Model file for the job. Use its own axes, mm. A direction names the side the tool comes from. Round coordinates to 2 decimals unless told otherwise and drop trailing zeros. Write each loop counter-clockwise with the first axis right and the second up, starting at its lowest first coordinate (ties: lowest second). Pieces come first, ordered by that corner, then holes. Notation, with made-up numbers: (52.5, -33.75) - (70.5, -33.75) arc R18 ccw to (70.5, -9.75) - close; hole circle Ø3 at (-1.75, 61.25). An arc over 180 degrees is marked (long way). Answer as a JSON object with one key per item and string values. Group by question number.
Autodesk Inventor part; units mm, degrees
ref_plane "YZ Plane" through (0, 0, 0) normal (1, 0, 0) x (0, 1, 0)
ref_plane "XZ Plane" through (0, 0, 0) normal (0, 1, 0) x (-1, 0, 0)
ref_plane "XY Plane" through (0, 0, 0) normal (0, 0, 1) x (1, 0, 0)
sketch "Sketch1" plane through (0, 0, 0) normal (0, 1, 0) x (-1, 0, 0)
  line L0 (-40, 30) -> (40, 30)
  line L1 (40, 30) -> (40, -30)
  line L2 (40, -30) -> (-40, -30)
  line L3 (-40, -30) -> (-40, 30)
  line L4 (-40, 30) -> (40, -30) construction
  line L5 (40, 30) -> (-40, -30) construction
  line L6 (25.245, -30) -> (20.245, -30)
  line L7 (20.245, 30) -> (25.245, 30)
  line L8 (37, 30) -> (37, -30)
  line L9 (30.9, -30) -> (30.9, 30)
  line L10 (25.9, -30) -> (25.9, 30)
  line L11 (-10.1, -30) -> (-10.1, 30) construction
  point P0 (0, 0)
  point P1 (-35, 20)
  point P2 (-35, -20)
  point P3 (-20.1, 20)
  point P4 (-20.1, -20)
  dimension "d0" = 80
  dimension "d1" = 60
  dimension "d3" = 3
  dimension "d4" = 6.1
  dimension "d5" = 5
  dimension "d6" = 10
  dimension "d7" = 10
  dimension "d8" = 5
  dimension "d9" = 5
  dimension "d10" = 36
  dimension "d11" = 10
  dimension "d12" = 10
extrude "Extrusion1" add sketch "Sketch1" along normal blind 5
extrude "Extrusion2" add sketch "Sketch1" along normal blind 15 contours L0 L9 L2 L10 | L0 L1 L2 L8
chamfer "Chamfer1" distance 1 angle 45 2 edges at (-37, 15, 0) (-30.9, 15, 0)
fillet "Fillet1" radius 5 1 edges at (-25.9, 5, 0)
hole "Hole1" at (35, 0, 20) at (35, 0, -20) at (20.1, 0, 20) at (20.1, 0, -20) direction (0, 1, 0) diameter 3 end through all countersink diameter 6 countersink angle 90
properties part number "stabilisateur"
(1) Slice it at C-C (z = 20). Write the cut outline in (x, y), then the cut area to 3 significant figures.
(2) Drill centre lines: line 1 (X direction, y = 3.05, z = -20); line 2 (Z direction, x = 35, y = 3.35); line 3 (X direction, y = 14, z = -7.5). Where is each one in solid material? Low to high. Write a range as from..to.
(3) Flat gauge pins, fed straight in: pin 1 (1.8 mm diameter, centred on x = 35, z = -20, fed in from +Y); pin 2 (4 mm diameter, centred on y = 13.5, z = 6, fed in from +X); pin 3 (2 mm diameter, centred on x = 15.5, z = -22, fed in from +Y); pin 4 (5 mm diameter, centred on x = -30.5, z = 5.5, fed in from +Y). Where does each tip first touch, or does it go through?
(4) 3-axis set-ups, long thin cutter, end or side, ignore diameter. For faces 4 (the flat face through (-30.9, 9, 0)), 5 (the flat face through (-39, 15, 0)): which of +Z, -Z, +X, -X, +Y, -Y reach the whole face in a straight line?
(5) Slice it at A-A (y = 12.5). Write the cut outline in (x, z).
(6) Pull direction X, two halves, no side cores. Call faces 1 (the flat face through (10, 5, 0)), 2 (the conical face through (35, 1, 18)), 3 (the flat face through (-25.9, 12, 0)): pulls with the +X half, pulls with the -X half, needs draft (parallel to the pull), parting line crosses it, or undercut.
(7) Slice it at B-B (x = 20.1). Write the cut outline in (y, z), then the cut area to 4 significant figures.
(8) Slice it at D-D (z = -25.5). Write the cut outline in (x, y), then the cut area to 3 significant figures.
Answer:
{
 "1": {"outline": "(-40, 0) - (17.1, 0) - (18.6, 1.5) - (18.6, 5) - (-20.9, 5) arc R5 cw to (-25.9, 10) - (-25.9, 15) - (-29.9, 15) - (-30.9, 14) - (-30.9, 5) - (-37, 5) - (-37, 14) - (-38, 15) - (-40, 15) - close; (21.6, 1.5) - (23.1, 0) - (32, 0) - (33.5, 1.5) - (33.5, 5) - (21.6, 5) - close; (36.5, 1.5) - (38, 0) - (40, 0) - (40, 5) - (36.5, 5) - close", "area": "450 mm²"},
 "2": {"line 1": "-40..18.6, 21.6..33.5, 36.5..40", "line 2": "-30..-21.5, -18.5..18.5, 21.5..30", "line 3": "-40..-37, -30.9..-25.9"},
 "3": {"pin 1": "through", "pin 2": "x = -25.9", "pin 3": "y = 5", "pin 4": "y = 15"},
 "4": {"face 4": "+Z, -Z, +Y", "face 5": "+Z, -Z, +X, -X, +Y"},
 "5": {"outline": "(-40, -30) - (-37, -30) - (-37, 30) - (-40, 30) - close; (-30.9, -30) - (-25.9, -30) - (-25.9, 30) - (-30.9, 30) - close"},
 "6": {"face 1": "needs draft", "face 2": "undercut", "face 3": "pulls with the +X half"},
 "7": {"outline": "(0, -30) - (5, -30) - (5, -21.5) - (1.5, -21.5) - (0, -23) - close; (0, -17) - (1.5, -18.5) - (5, -18.5) - (5, 18.5) - (1.5, 18.5) - (0, 17) - close; (0, 23) - (1.5, 21.5) - (5, 21.5) - (5, 30) - (0, 30) - close", "area": "265.5 mm²"},
 "8": {"outline": "(-40, 0) - (40, 0) - (40, 5) - (-20.9, 5) arc R5 cw to (-25.9, 10) - (-25.9, 15) - (-29.9, 15) - (-30.9, 14) - (-30.9, 5) - (-37, 5) - (-37, 14) - (-38, 15) - (-40, 15) - close", "area": "484 mm²"}
}
